Autodesk Inventor part; units mm, degrees
ref_plane "YZ Plane" through (0, 0, 0) normal (1, 0, 0) x (0, 1, 0)
ref_plane "XZ Plane" through (0, 0, 0) normal (0, 1, 0) x (-1, 0, 0)
ref_plane "XY Plane" through (0, 0, 0) normal (0, 0, 1) x (1, 0, 0)
sketch "スケッチ1" plane through (0, 0, 0) normal (0, 0, 1) x (1, 0, 0)
  circle A0 centre (0, 0) radius 27.5
  line L0 (0, 27.5) -> (0, 0)
  line L1 (8, 0) -> (19.445271, -19.445602)
  line L2 (0, 0) -> (27.5, 0)
  circle A1 centre (19.445271, -19.445602) radius 5
  circle A2 centre (0, 0) radius 10
  arc A3 (24.316088, -20.574825) -> (0, 10.000005) centre (0.018653, -14.941839) ccw
  line L3 (24.316088, -20.574825) -> (14.574455, -20.574825)
  arc A4 (14.574455, -20.574825) -> (0.517924, -9.986579) centre (1.227526, -23.669106) ccw
  arc A5 (-24.316088, 20.574825) -> (0, -10.000005) centre (-0.018653, 14.941839) ccw
  arc A6 (-14.574455, 20.574825) -> (-0.517924, 9.986579) centre (-1.227526, 23.669106) ccw
  circle A7 centre (-19.445271, 19.445602) radius 5
  point P0 (-0.517924, 9.986579)
  point P1 (0, -10)
  point P2 (0, 10.000005)
  dimension "d4" = 20
  dimension "d0" = 55
  dimension "d1" = 8
  dimension "d2" = 22.56381
  dimension "d3" = 10
  dimension "d5" = 9.74163
  dimension "d9" = 360
sketch "スケッチ1 outline for 押し出し1" plane through (0, 0, 0) normal (0, 0, 1) x (1, 0, 0)
  arc A0 (14.574455, -20.574825) -> (24.316088, -20.574825) centre (19.445271, -19.445602) ccw
  arc A1 (24.316088, -20.574825) -> (0, 10.000005) centre (0.018653, -14.941839) ccw
  arc A2 (0, 10) -> (-0.517924, 9.986579) centre (0, 0) ccw
  arc A3 (-0.517924, 9.986579) -> (-14.574455, 20.574825) centre (-1.227526, 23.669106) cw
  arc A4 (-14.574455, 20.574825) -> (-24.316088, 20.574825) centre (-19.445271, 19.445602) ccw
  arc A5 (-24.316088, 20.574825) -> (0, -10) centre (-0.018659, 14.941837) ccw
  arc A6 (0, -10) -> (0.517924, -9.986579) centre (0, 0) ccw
  arc A7 (0.517924, -9.986579) -> (14.574455, -20.574825) centre (1.227526, -23.669106) cw
extrude "押し出し1" add sketch "スケッチ1 outline for 押し出し1" along normal blind 3
sketch "スケッチ2" plane through (0, 0, 3) normal (0, 0, 1) x (1, 0, 0)
  circle A0 centre (0, 0) radius 4.25
  dimension "d13" = 8.5
extrude "押し出し2" cut sketch "スケッチ2" against normal blind 3
sketch "スケッチ3" plane through (0, 0, 3) normal (0, 0, 1) x (1, 0, 0)
  arc A0 (-14.574455, 20.574825) -> (-24.316088, 20.574825) centre (-19.445271, 19.445602) ccw
  arc A1 (14.574455, -20.574825) -> (24.316088, -20.574825) centre (19.445271, -19.445602) ccw
  circle A2 centre (0, 0) radius 4.25
  point P0 (8, 0)
  point P1 (-8, 0)
  point P2 (0, 8)
  point P3 (-8, 0)
  point P4 (0, -8)
  dimension "d16" = 8
  dimension "d17" = 8
  dimension "d49" = 360
hole "穴1" at (-19.445271, 19.445602, 3) at (19.445271, -19.445602, 3) at (8, 0, 3) at (-8, 0, 3) at (0, 8, 3) at (0, -8, 3) direction (0, 0, -1) diameter 2 end through all
sketch "スケッチ4" plane through (0, 0, 3) normal (0, 0, 1) x (1, 0, 0)
  circle A0 centre (0, 0) radius 9.289
  circle A1 centre (8, 0) radius 1
  circle A2 centre (8, 0) radius 6.227
  circle A3 centre (0, 0) radius 8.107
  circle A4 centre (8, 0) radius 4.267399
  line L0 (6.969375, 6.141119) -> (6.969547, 4.141119)
  circle A5 centre (6.970301, -6.696881) radius 12.838
  circle A6 centre (0, 0) radius 20.909
  circle A7 centre (8, 0) radius 13.574
  line L1 (19.8083, -6.694589) -> (17.8083, -6.694761)
  arc A8 (17.8083, -6.694761) -> (6.969547, 4.141119) centre (6.970301, -6.696881) ccw
  circle A9 centre (-6.970301, 6.696881) radius 12.838
  line L2 (-19.8083, 6.694589) -> (-17.8083, 6.694761)
  arc A10 (-17.8083, 6.694761) -> (-6.969547, -4.141119) centre (-6.970301, 6.696881) ccw
  line L3 (-6.969375, -6.141119) -> (-6.969547, -4.141119)
  point P0 (6.969547, 4.141119)
  point P1 (-6.969547, -4.141119)
  dimension "d25" = 18.578
  dimension "d26" = 12.454
  dimension "d30" = 41.818
  dimension "d31" = 27.148
  dimension "d27" = 16.214
  dimension "d29" = 25.676
  dimension "d32" = 2
  dimension "d33" = 2
  dimension "d36" = 360
extrude "押し出し3" add sketch "スケッチ4" along normal blind 2 contours A8 A4 A0 | A0 A4 A8 | A4 L0 A0 | A0 A5 A2 A8 A4 | A2 A5 L1 A8 | A9 L2 A10 A0 | A0 A10 L3 picked at (7.717949, 4.165451) picked at (9.179473, 4.022297)
sketch "スケッチ5" plane through (0, 0, 0) normal (0, 0, -1) x (-1, 0, 0)
  circle A0 centre (19.445271, 19.445602) radius 1
  circle A1 centre (-19.445271, -19.445602) radius 1
  point P0 (0, 0)
hole "穴2" at (-19.445271, 19.445602, 0) at (19.445271, -19.445602, 0) direction (0, 0, 1) diameter 3.1 end through all
properties part number "rotor" material "アルミニウム 6061"
CAD build for the part. Positions are in the model's coordinates, mm. A direction names the side the tool comes from. Coordinates: 2 decimals unless noted, no trailing zeros. Order: outer loops, then holes, each group sorted by start corner. A loop starts at its lowest first (then second) coordinate and runs counter-clockwise, first axis right, second up. Notation, with made-up numbers: (-29, 52) -> (20, 52) arc R15 cw to (20, 63) -> close; hole circle Ø4 at (27.25, 25.5). An arc over 180 degrees is marked (long way). Use one line per item in the form item = value. Start each with the question number.
1) Band-saw the part on C-C on y = -8. Give the cut face in (x, z) (3 decimals), then the cut area to 3 significant figures.
2) Band-saw the part on D-D on z = 0.95. Give the cut face in (x, y), then the cut area to 3 significant figures.
3) Band-saw the part on A-A on z = 4.3. Give the cut face in (x, y).
4) Pull direction Y, two halves, no side cores. Call faces 4 (the cylindrical face through (-18.502, 18.216, 1.521)), 5 (the cylindrical face through (17.91, -19.65, 1.52)), 6 (the cylindrical face through (-19.539, 24.445, 1.479)), 7 (the cylindrical face through (14.5, 1.1, 4)): +Y half, -Y half, draft (parallel to the pull), parting line (faces both ways), or undercut.
5) Drill centre lines: L1, parallel to Y at x = 0, z = 1.6; L2, parallel to Z at x = 14, y = -2; L3, parallel to Y at x = 8, z = 1.2. Where is each one in solid material? Low to high. Write a range as [from, to].
6) Drop flat-ended pins along their axis: pin 1 (2 mm diameter, centred on x = 19, z = 2.5, fed in from +Y); pin 2 (1 mm diameter, centred on y = 17, z = 1, fed in from -X); pin 3 (1.2 mm diameter, centred on x = 0, y = -8, fed in from +Z); pin 4 (1.6 mm diameter, centred on y = 5, z = 4, fed in from -X). Give the stop position or say it passes through.
7) Band-saw the part on B-B on x = 8. Give the cut face in (y, z).
8) Tool access for faces 1 (the cylindrical face through (-14.5, -1.1, 4)), 2 (the cylindrical face through (0.6, -7.2, 1.5)), 3 (the cylindrical face through (-15.95, -2.48, 3.99)): list every direction of +Z, -Z, +X, -X, +Y, -Y with a clear straight run to the whole face (end or side of a thin tool).
Entries:
q1.outline = (-9.805, 0) -> (-1, 0) -> (-1, 3) -> (-9.805, 3) -> close; (1, 0) -> (23.975, 0) -> (23.975, 3) -> (1, 3) -> close
q1.area = 95.3 mm2
q2.outline = (-24.32, 20.57) arc R24.94 ccw to (0, -10) arc R10 ccw to (0.52, -9.99) arc R13.7 cw to (14.57, -20.57) arc R5 ccw to (24.32, -20.57) arc R24.94 ccw to (0, 10) arc R10.01 ccw to (-0.52, 9.99) arc R13.7 cw to (-14.57, 20.57) arc R5 ccw to start; hole circle Ø3.1 at (-19.45, 19.45); hole circle Ø2 at (-8, 0); hole circle Ø8.5 at (0, 0); hole circle Ø2 at (0, -8); hole circle Ø2 at (0, 8); hole circle Ø2 at (8, 0); hole circle Ø3.1 at (19.45, -19.45)
q2.area = 992 mm2
q3.outline = (-19.81, 6.69) arc R12.84 ccw to (-6.97, -6.14) -> (-6.97, -4.14) arc R10.84 cw to (-17.81, 6.69) -> close; (6.97, 4.14) arc R10.84 cw to (17.81, -6.69) -> (19.81, -6.69) arc R12.84 ccw to (6.97, 6.14) -> close
q4.face_4 = undercut
q4.face_5 = undercut
q4.face_6 = +Y half
q4.face_7 = -Y half
q5.L1 = [-10, -9], [-7, -4.25], [4.25, 7], [9, 10]
q5.L2 = [0, 3]
q5.L3 = [-11.76, -1], [1, 8.69]
q6.pin_1 = 2.34
q6.pin_2 = -24.91
q6.pin_3 = through
q6.pin_4 = -19.78
q7.outline = (-11.76, 0) -> (-1, 0) -> (-1, 3) -> (-11.76, 3) -> close; (1, 0) -> (8.69, 0) -> (8.69, 3) -> (6.1, 3) -> (6.1, 5) -> (4.09, 5) -> (4.09, 3) -> (1, 3) -> close
q8.face_1 = +Z, +Y
q8.face_2 = +Z, -Z
q8.face_3 = +Z, -X, -Y
